The model under review builds one solid part; all positions refer to its coordinate system, in mm. Face numbers are marked on the shaded views. A direction names the side the tool comes from. Give positions to 0.01 mm unless a question says otherwise; leave off trailing zeros. Loops run counter-clockwise (first coordinate to the right, second up) from the corner with the lowest first, then second, coordinate; pieces in that order, holes last. Notation, with made-up numbers: M -13,41.25 L 15,41.25 A18 cw 15,69.25 Z; hole C 31,-33 d5. An arc over 180 degrees is marked long. Return JSON: item names as keys, results as strings.
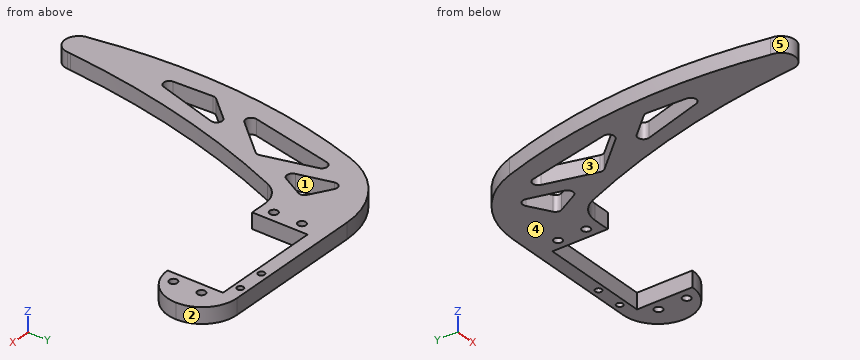
```python
from build123d import *

# Parameters (mm, degrees)
BOSS_EXTRU_1_DEPTH      = 5.66
ENL_V_MAT_EXTRU_1_REACH = 135.062
ESQUISSE2_W             = 40
ESQUISSE2_H             = 20
ENL_V_MAT_EXTRU_2_REACH = 135.062
ESQUISSE3_R             = 1.45
CONG_2_R                = 12.5
CONG_3_R                = 10
CONG_4_R                = 30
CONG_5_R                = 30
ENL_V_MAT_EXTRU_3_REACH = 135.062
CONG_6_R                = 2
ENL_V_MAT_EXTRU_4_REACH = 135.062
ESQUISSE5_R             = 1.15


# Some blends are built 0.0001 mm under size
with BuildPart() as part:
    # Esquisse1 → Boss.-Extru.1 (new body)
    with BuildSketch(Plane.XY):
        with BuildLine():
            Line((-32.5, 12.5), (-52.5, 12.5))
            ThreePointArc((-52.5, 12.5), (-69.287355537, -46.339080558), (-67.5, -107.5))
            ThreePointArc((-67.5, -107.5), (-62.5, -112.5), (-57.5, -107.5))
            ThreePointArc((-57.5, -107.5), (-48.914858734, -58.969774017), (-32.5, -12.5))
            Line((-32.5, -12.5), (32.5, -12.5))
            Line((32.5, -12.5), (32.5, 12.5))
            Line((32.5, 12.5), (-32.5, 12.5))
        make_face()
    extrude(amount=BOSS_EXTRU_1_DEPTH)

    # Esquisse2 → Enlèv. mat.-Extru.1 (cut, up to next)
    with BuildSketch(Plane.XY.offset(5.66), mode=Mode.PRIVATE) as enl_v_mat_extru_1_sk1:
        with Locations((0, -2.5)):
            Rectangle(ESQUISSE2_W, ESQUISSE2_H)
    enl_v_mat_extru_1_tool1 = extrude(enl_v_mat_extru_1_sk1.sketch, amount=-ENL_V_MAT_EXTRU_1_REACH, mode=Mode.PRIVATE) & part.part
    add(enl_v_mat_extru_1_tool1.solids().sort_by_distance((0, -2.5, 5.66))[0], mode=Mode.SUBTRACT)

    # Esquisse3 → Enlèv. mat.-Extru.2 (cut, up to next)
    with BuildSketch(Plane.XY.offset(5.66), mode=Mode.PRIVATE) as enl_v_mat_extru_2_sk1:
        with Locations((-23.75, -7.58)):
            Circle(ESQUISSE3_R)
    enl_v_mat_extru_2_tool1 = extrude(enl_v_mat_extru_2_sk1.sketch, amount=-ENL_V_MAT_EXTRU_2_REACH, mode=Mode.PRIVATE) & part.part
    # Esquisse3 → Enlèv. mat.-Extru.2 (cut, up to next)
    with BuildSketch(Plane.XY.offset(5.66), mode=Mode.PRIVATE) as enl_v_mat_extru_2_sk2:
        with Locations((23.75, -7.58)):
            Circle(ESQUISSE3_R)
    enl_v_mat_extru_2_tool2 = extrude(enl_v_mat_extru_2_sk2.sketch, amount=-ENL_V_MAT_EXTRU_2_REACH, mode=Mode.PRIVATE) & part.part
    # Esquisse3 → Enlèv. mat.-Extru.2 (cut, up to next)
    with BuildSketch(Plane.XY.offset(5.66), mode=Mode.PRIVATE) as enl_v_mat_extru_2_sk3:
        with Locations((23.75, 2.58)):
            Circle(ESQUISSE3_R)
    enl_v_mat_extru_2_tool3 = extrude(enl_v_mat_extru_2_sk3.sketch, amount=-ENL_V_MAT_EXTRU_2_REACH, mode=Mode.PRIVATE) & part.part
    # Esquisse3 → Enlèv. mat.-Extru.2 (cut, up to next)
    with BuildSketch(Plane.XY.offset(5.66), mode=Mode.PRIVATE) as enl_v_mat_extru_2_sk4:
        with Locations((-23.75, 2.58)):
            Circle(ESQUISSE3_R)
    enl_v_mat_extru_2_tool4 = extrude(enl_v_mat_extru_2_sk4.sketch, amount=-ENL_V_MAT_EXTRU_2_REACH, mode=Mode.PRIVATE) & part.part
    add(enl_v_mat_extru_2_tool1.solids().sort_by_distance((-23.75, -7.58, 5.66))[0], mode=Mode.SUBTRACT)
    add(enl_v_mat_extru_2_tool2.solids().sort_by_distance((23.75, -7.58, 5.66))[0], mode=Mode.SUBTRACT)
    add(enl_v_mat_extru_2_tool3.solids().sort_by_distance((23.75, 2.58, 5.66))[0], mode=Mode.SUBTRACT)
    add(enl_v_mat_extru_2_tool4.solids().sort_by_distance((-23.75, 2.58, 5.66))[0], mode=Mode.SUBTRACT)

    # Congé2
    cong_2_edges = [part.edges().sort_by_distance(p)[0] for p in [
        (32.5, -12.5, 2.83),
        (32.5, 12.5, 2.83),
    ]]
    fillet(cong_2_edges, radius=CONG_2_R - 0.0001)  # a hair under: the kernel refuses the full size

    # Congé3
    cong_3_edges = [part.edges().sort_by_distance(p)[0] for p in [
        (-32.5, -12.5, 2.83),
    ]]
    fillet(cong_3_edges, radius=CONG_3_R)

    # Congé4
    cong_4_edges = [part.edges().sort_by_distance(p)[0] for p in [
        (-52.5, 12.5, 2.83),
    ]]
    fillet(cong_4_edges, radius=CONG_4_R)

    # Congé5
    # the kernel refuses this fillet: 30 mm, written as the material it adds along each edge
    with BuildSketch(Plane(origin=(-57.5, -107.5, 0), x_dir=(-0.029294676062998543, -0.9995708188789647, 0), z_dir=(0, 0, 1))) as cong_5_piece_1:
        with BuildLine():
            CenterArc((1.171787043, 29.987124566), CONG_5_R, 266.202223448, 2.119075089)
            ThreePointArc((-0.815268333, 0.053003384), (-0.407652209, 0.026224165), (0, 0))
            ThreePointArc((0, 0), (0.14647338, 0.002145906), (0.292946761, 0))
        make_face()
    extrude(amount=5.66)

    # Esquisse4 → Enlèv. mat.-Extru.3 (cut, up to next)
    with BuildSketch(Plane.XY.offset(5.66), mode=Mode.PRIVATE) as enl_v_mat_extru_3_sk1:
        Polygon((-35.530484253, -6.741676359), (-42.974151572, -20.332321303), (-48.555833289, 0.989708193), align=None)
    enl_v_mat_extru_3_tool1 = extrude(enl_v_mat_extru_3_sk1.sketch, amount=-ENL_V_MAT_EXTRU_3_REACH, mode=Mode.PRIVATE) & part.part
    # Esquisse4 → Enlèv. mat.-Extru.3 (cut, up to next)
    with BuildSketch(Plane.XY.offset(5.66), mode=Mode.PRIVATE) as enl_v_mat_extru_3_sk2:
        Polygon((-52.982896502, -3.816878406), (-45.919055028, -30.800759586), (-62.900626013, -49.913479621), align=None)
    enl_v_mat_extru_3_tool2 = extrude(enl_v_mat_extru_3_sk2.sketch, amount=-ENL_V_MAT_EXTRU_3_REACH, mode=Mode.PRIVATE) & part.part
    # Esquisse4 → Enlèv. mat.-Extru.3 (cut, up to next)
    with BuildSketch(Plane.XY.offset(5.66), mode=Mode.PRIVATE) as enl_v_mat_extru_3_sk3:
        Polygon((-49.898192375, -43.559912364), (-63.702500518, -59.0966302), (-62.552958266, -85.696486809), align=None)
    enl_v_mat_extru_3_tool3 = extrude(enl_v_mat_extru_3_sk3.sketch, amount=-ENL_V_MAT_EXTRU_3_REACH, mode=Mode.PRIVATE) & part.part
    add(enl_v_mat_extru_3_tool1.solids().sort_by_distance((-42.35349, -8.694763, 5.66))[0], mode=Mode.SUBTRACT)
    add(enl_v_mat_extru_3_tool2.solids().sort_by_distance((-53.934193, -28.177039, 5.66))[0], mode=Mode.SUBTRACT)
    add(enl_v_mat_extru_3_tool3.solids().sort_by_distance((-58.717884, -62.784343, 5.66))[0], mode=Mode.SUBTRACT)

    # Congé6
    cong_6_edges = [part.edges().sort_by_distance(p)[0] for p in [
        (-62.900626013, -49.913479621, 2.83),
        (-52.982896502, -3.816878406, 2.83),
        (-45.919055028, -30.800759586, 2.83),
        (-49.898192375, -43.559912364, 2.83),
        (-62.552958266, -85.696486809, 2.83),
        (-63.702500518, -59.0966302, 2.83),
        (-48.555833289, 0.989708193, 2.83),
        (-35.530484253, -6.741676359, 2.83),
        (-42.974151572, -20.332321303, 2.83),
    ]]
    fillet(cong_6_edges, radius=CONG_6_R)

    # Esquisse5 → Enlèv. mat.-Extru.4 (cut, up to next)
    with BuildSketch(Plane.XY.offset(5.66), mode=Mode.PRIVATE) as enl_v_mat_extru_4_sk1:
        with Locations((15, 9.91)):
            Circle(ESQUISSE5_R)
    enl_v_mat_extru_4_tool1 = extrude(enl_v_mat_extru_4_sk1.sketch, amount=-ENL_V_MAT_EXTRU_4_REACH, mode=Mode.PRIVATE) & part.part
    # Esquisse5 → Enlèv. mat.-Extru.4 (cut, up to next)
    with BuildSketch(Plane.XY.offset(5.66), mode=Mode.PRIVATE) as enl_v_mat_extru_4_sk2:
        with Locations((5, 9.91)):
            Circle(ESQUISSE5_R)
    enl_v_mat_extru_4_tool2 = extrude(enl_v_mat_extru_4_sk2.sketch, amount=-ENL_V_MAT_EXTRU_4_REACH, mode=Mode.PRIVATE) & part.part
    add(enl_v_mat_extru_4_tool1.solids().sort_by_distance((15, 9.91, 5.66))[0], mode=Mode.SUBTRACT)
    add(enl_v_mat_extru_4_tool2.solids().sort_by_distance((5, 9.91, 5.66))[0], mode=Mode.SUBTRACT)


solid = part.part
```
1) Wall thickness on L1, parallel to Y at x = -23.75, z = 2.3; L2, parallel to Y at x = -23.5, z = 0.85; L3, parallel to X at y = -2.5, z = 2.1: over which ranges is each line inside the solid? List them lowest first. Write a range as from..to.
From the geometry:
{"L1": "-12.5..-9.03, -6.13..1.13, 4.03..12.5", "L2": "-12.5..-9.01, -6.15..1.15, 4.01..12.5", "L3": "-58.13..-47.25, -42.68..-20, 20..32.25"}
2) Consider section A-A on y = -62.5. Write out the cut boundary in (x, z).
From the geometry:
{"outline": "M -70.64,0 L -63.56,0 L -63.56,5.66 L -70.64,5.66 Z; M -55.59,0 L -49.82,0 L -49.82,5.66 L -55.59,5.66 Z"}
3) The part is to be moulded in two halves that separate along Y. For the marked faces 3, 4 and 5, say which applies: released by +Y, released by -Y, zero draft, split by the parting line, or undercut.
From the geometry:
{"face 3": "undercut", "face 4": "zero draft", "face 5": "released by -Y"}
4) Tool access review of the marked faces 1 and 2: name each direction out of +Z, -Z, +X, -X, +Y, -Y from which nothing blocks a thin tool from reaching the whole face with its end or side.
From the geometry:
{"face 1": "+Z, -Z", "face 2": "+Z, -Z, +X, +Y"}
5) Insertion check: pin 1 (1.7 mm diameter, centred on x = -22.5, z = 3.5, fed in from -Y); pin 2 (3 mm diameter, centred on y = -4, z = 4, fed in from +X); pin 3 (1 mm diameter, centred on y = -4, z = 3, fed in from -X). Each pin has a flat end and moves straight along its axis. Give the tip position at first contact, or say it passes through.
From the geometry:
{"pin 1": "y = -12.5", "pin 2": "x = 32.25", "pin 3": "x = -59.18"}
6) Consider section B-B on z = 2.45. Count the separate pieces of the cut face and the enclosed holes in it, then the cut area to 3 significant figures.
From the geometry:
{"separate pieces": "1", "enclosed holes": "9", "area": "2,750 mm²"}
7) Consider section D-D on y = -26.5. Write out the cut boundary in (x, z), then the cut area to 3 significant figures.
From the geometry:
{"outline": "M -65.78,0 L -57.86,0 L -57.86,5.66 L -65.78,5.66 Z; M -47.04,0 L -38.36,0 L -38.36,5.66 L -47.04,5.66 Z", "area": "94.0 mm²"}
8) Consider section C-C on x = -4. Write out the cut boundary in (y, z), then the cut area to 3 significant figures.
From the geometry:
{"outline": "M 7.5,0 L 12.5,0 L 12.5,5.66 L 7.5,5.66 Z", "area": "28.3 mm²"}
